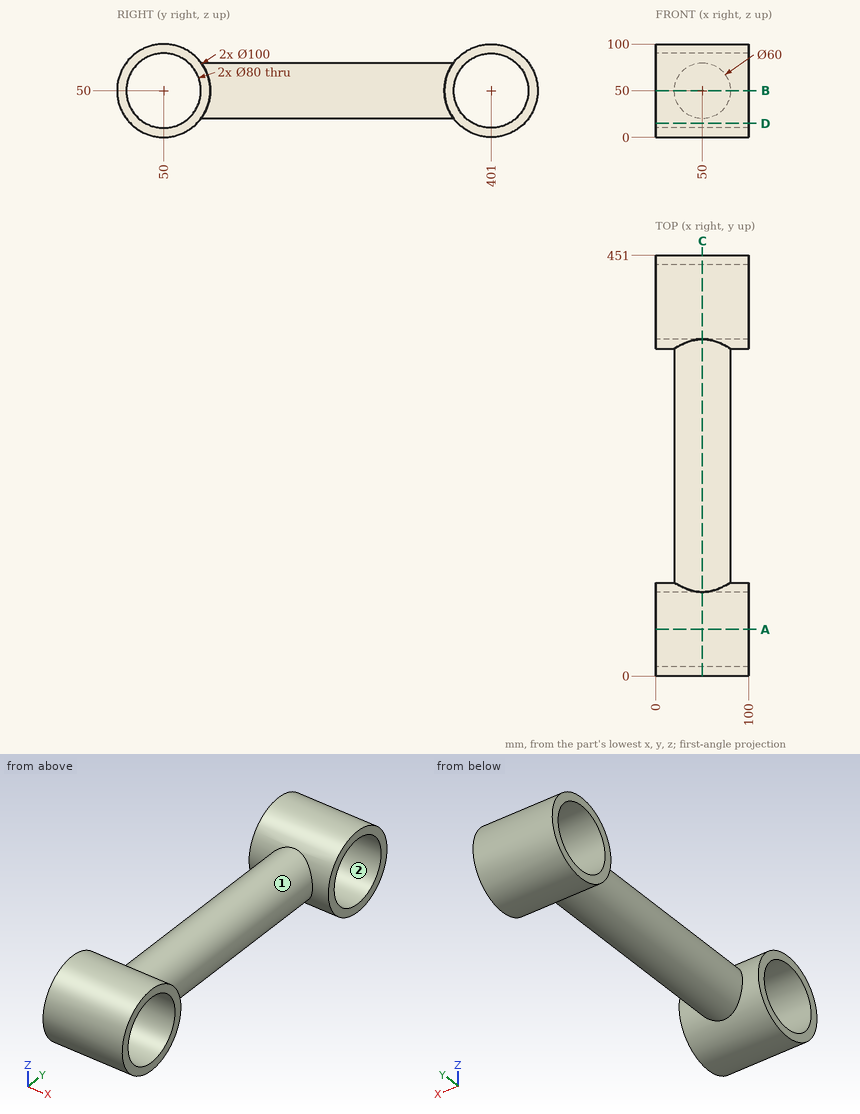
Job drawing, mm, ordinate dimensions from the low corner. One solid piece. A direction names the side the tool comes from. Round coordinates to 2 decimals unless told otherwise and drop trailing zeros. Loops run counter-clockwise (first coordinate to the right, second up) from the corner with the lowest first, then second, coordinate; pieces in that order, holes last.
(1) Drop flat-ended pins along their axis: pin 1 (1.5 mm diameter, centred on x = 20.5, y = 53.5, fed in from -Z); pin 2 (1.5 mm diameter, centred on y = 114.5, z = 71.5, fed in from -X); pin 3 (5 mm diameter, centred on y = 133.5, z = 47.5, fed in from -X). Give the stop position or say it passes through.
(2) Cut at C-C (x = 50). Give the cut face in (y, z), plus the area to 3 significant figures.
(3) Cut at A-A (y = 50). Give the cut face in (x, z), plus the area to 3 significant figures.
(4) Which spindle directions (+Z, -Z, +X, -X, +Y, -Y) get a long thin tool onto all of the face, cutting with end or side? Do the marked faces 1 and 2. Say none if no direction does.
(5) Wall check: line 1 along Y through (x, z) = (71, 50); line 2 along Y through (x, z) = (6.5, 36); line 3 along Y through (x, z) = (77, 72). Give the ranges that are in metal, low to high.
(6) Cut at B-B (z = 50). Give the cut face in (x, y), plus the area to 3 significant figures.
(7) Cut at D-D (z = 15). Give the cut face in (x, y), plus the area to 3 significant figures.
Findings below:
1. pin 1: stops at z = 0.08
1. pin 2: stops at x = 28.33
1. pin 3: stops at x = 20
2. outline: (90, 20) - (361, 20) arc R50 ccw (long way) to (361, 80) - (90, 80) arc R50 ccw (long way) to start; hole circle Ø80 at (50, 50); hole circle Ø80 at (401, 50)
2. area: 21,100 mm2
3. outline: (0, 0) - (100, 0) - (100, 10) - (0, 10) - close; (0, 90) - (100, 90) - (100, 100) - (0, 100) - close
3. area: 2,000 mm2
4. face 1: none
4. face 2: +X, -X
5. line 1: y = 0 to 10, 90 to 361, 441 to 451
5. line 2: y = 2 to 12.53, 87.47 to 98, 353 to 363.53, 438.47 to 449
5. line 3: y = 5.1 to 16.59, 83.41 to 94.9, 356.1 to 367.59, 434.41 to 445.9
6. outline: (0, 0) - (100, 0) - (100, 10) - (0, 10) - close; (0, 90) - (100, 90) - (100, 100) - (80, 100) - (80, 351) - (100, 351) - (100, 361) - (0, 361) - (0, 351) - (20, 351) - (20, 100) - (0, 100) - close; (0, 441) - (100, 441) - (100, 451) - (0, 451) - close
6. area: 19,100 mm2
7. outline: (0, 14.29) - (100, 14.29) - (100, 30.64) - (0, 30.64) - close; (0, 69.36) - (100, 69.36) - (100, 85.71) - (0, 85.71) - close; (0, 365.29) - (100, 365.29) - (100, 381.64) - (0, 381.64) - close; (0, 420.36) - (100, 420.36) - (100, 436.71) - (0, 436.71) - close
7. area: 6,540 mm2
